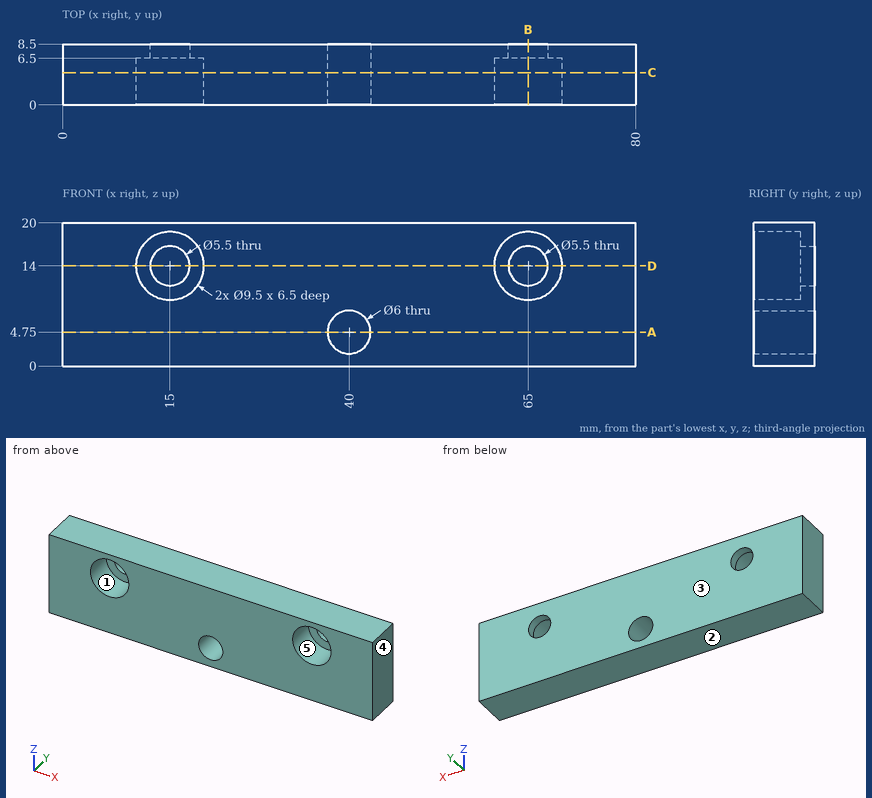
The figure shows three views and two pictorial views of one solid part (mm, origin at its lowest corner). Answer the questions. A direction names the side the tool comes from. Give positions to 0.01 mm unless a question says otherwise; leave off trailing zeros. Write each loop counter-clockwise with the first axis right and the second up, starting at its lowest first coordinate (ties: lowest second). Pieces come first, ordered by that corner, then holes.
Q1. The part is cut by section C-C on y = 4.5. Give the vertices of the cut face in (x, z), and give its area (3 significant figures).
Answer:
outline: (0, 0) - (80, 0) - (80, 20) - (0, 20) - close; hole circle Ø9.5 at (15, 14); hole circle Ø6 at (40, 4.75); hole circle Ø9.5 at (65, 14)
area: 1,430 mm2
Q2. A tool of negligible diameter and unlimited length cuts with its end or side. For the marked faces 4 and 5, from which of +Z, -Z, +X, -X, +Y, -Y can it reach the whole face along a straight path? Write none if from no direction.
Answer:
face 4: +Z, -Z, +X, +Y, -Y
face 5: -Y
Q3. Straight lines are drawn through the part: L1, parallel to Z at x = 15, y = 3; L2, parallel to Z at x = 15, y = 7.2; L3, parallel to X at y = 5.5, z = 5.25. For each, find the intervals that lie inside material, in ascending order.
Answer:
L1: z = 0 to 9.25, 18.75 to 20
L2: z = 0 to 11.25, 16.75 to 20
L3: x = 0 to 37.04, 42.96 to 80
Q4. Given pin 1 (4 mm diameter, centred on x = 16.5, z = 13, fed in from -Y), flat-ended and moving along its own axis, determine where the tip first touches the part or whether it passes through.
Answer:
pin 1: stops at y = 6.5
Q5. The part is cut by section D-D on z = 14. Give the vertices of the cut face in (x, y), and give its area (4 significant figures).
Answer:
outline: (0, 0) - (10.25, 0) - (10.25, 6.5) - (12.25, 6.5) - (12.25, 8.5) - (0, 8.5) - close; (17.75, 6.5) - (19.75, 6.5) - (19.75, 0) - (60.25, 0) - (60.25, 6.5) - (62.25, 6.5) - (62.25, 8.5) - (17.75, 8.5) - close; (67.75, 6.5) - (69.75, 6.5) - (69.75, 0) - (80, 0) - (80, 8.5) - (67.75, 8.5) - close
area: 534.5 mm2
Q6. For a pull along Z with two mould halves and no side action, classify the marked faces 1, 2 and 3 as released by +Z, released by -Z, zero draft, split by the parting line, or undercut.
Answer:
face 1: undercut
face 2: released by -Z
face 3: zero draft
Q7. The part is cut by section B-B on x = 65. Give the vertices of the cut face in (y, z).
Answer:
outline: (0, 0) - (8.5, 0) - (8.5, 11.25) - (6.5, 11.25) - (6.5, 9.25) - (0, 9.25) - close; (0, 18.75) - (6.5, 18.75) - (6.5, 16.75) - (8.5, 16.75) - (8.5, 20) - (0, 20) - close
Q8. The part is cut by section A-A on z = 4.75. Give the vertices of the cut face in (x, y), and give its area (3 significant figures).
Answer:
outline: (0, 0) - (37, 0) - (37, 8.5) - (0, 8.5) - close; (43, 0) - (80, 0) - (80, 8.5) - (43, 8.5) - close
area: 629 mm2
